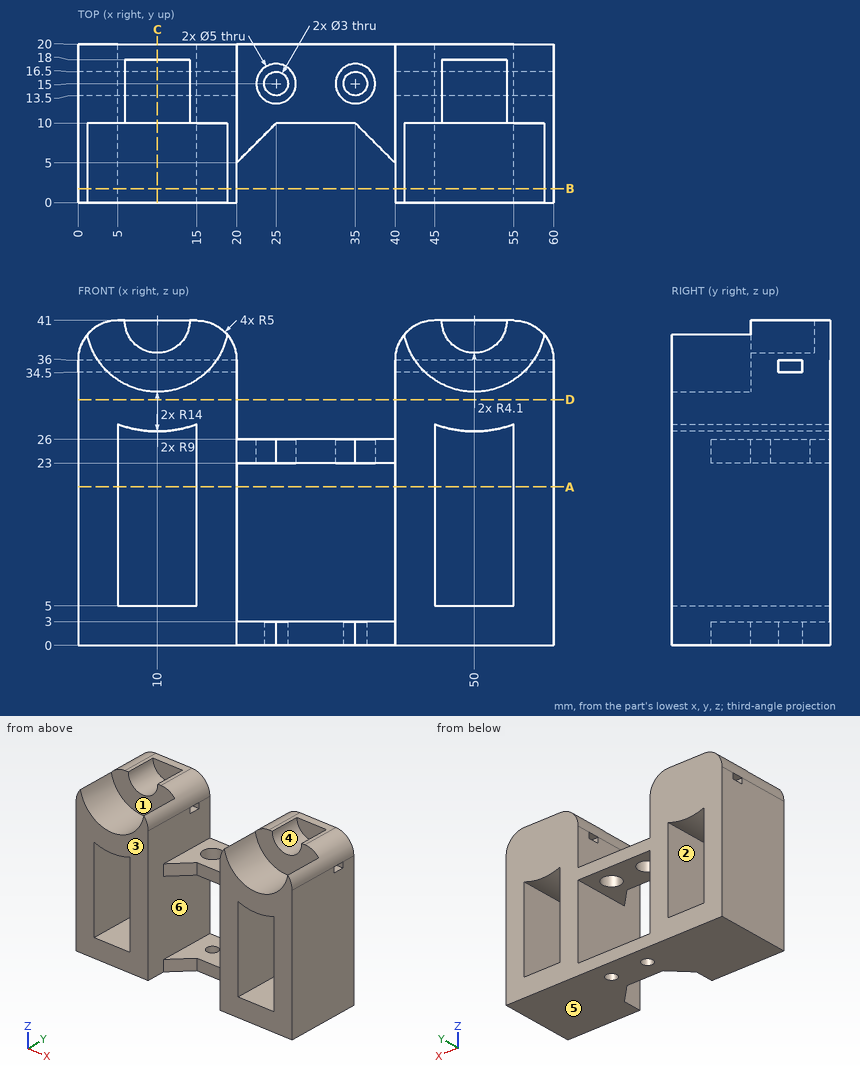
Check sheet for the drawn part. Datum: minimum x, y, z corner. Units: mm. A direction names the side the tool comes from. Round coordinates to 2 decimals unless told otherwise and drop trailing zeros. Loops run counter-clockwise (first coordinate to the right, second up) from the corner with the lowest first, then second, coordinate; pieces in that order, holes last. Notation, with made-up numbers: (71, 24.25) -> (80, 24.25) arc R23 ccw to (80, 57.25) -> close; hole circle Ø10 at (-35, -40). An arc over 180 degrees is marked (long way). Put each result on its own line as item: value. Start each with the question number.
1. Section check B-B (y = 1.75). Enter the section's corners in (x, z).
2. Section check D-D (z = 31). Enter the section's corners in (x, y).
3. Section check C-C (x = 10). Enter the section's corners in (y, z).
4. Gauge pin test, flat ends, axial feed: pin 1 (6 mm diameter, centred on x = 12, z = 28, fed in from -Y); pin 2 (3.5 mm diameter, centred on x = 32, z = 25, fed in from -Y); pin 3 (6.5 mm diameter, centred on x = 35, y = 15, fed in from +Z); pin 4 (1.2 mm diameter, centred on x = 10, z = 40, fed in from -Y). Record the tip position at first contact, or that the pin passes through.
5. Scan lines: probe 1 along X at (y, z) = (6.25, 15); probe 2 along Z at (x, y) = (39.5, 15.5); probe 3 along X at (y, z) = (8.25, 29). Record each from-to range of solid material in increasing order.
6. Section check A-A (z = 20). Enter the section's corners in (x, y), plus the area to 3 significant figures.
7. Access from +Z, -Z, +X, -X, +Y, -Y to the whole of each face (thin tool, end or side, straight path). Record for the marked faces 1, 2 and 3.
8. Draft check along Z on the marked faces 4, 5 and 6. Enter one of: +Z half, -Z half, draft (parallel to the pull), parting line (faces both ways), or undercut.
Findings:
1. outline: (0, 0) -> (20, 0) -> (20, 36) arc R5 ccw to (18.82, 39.22) arc R9 cw to (1.18, 39.22) arc R5 ccw to (0, 36) -> close; (40, 0) -> (60, 0) -> (60, 36) arc R5 ccw to (58.82, 39.22) arc R9 cw to (41.18, 39.22) arc R5 ccw to (40, 36) -> close; hole (5, 5) -> (15, 5) -> (15, 27.92) arc R14 cw to (5, 27.92) -> close; hole (45, 5) -> (55, 5) -> (55, 27.92) arc R14 cw to (45, 27.92) -> close
2. outline: (0, 0) -> (20, 0) -> (20, 20) -> (0, 20) -> close; (40, 0) -> (60, 0) -> (60, 20) -> (40, 20) -> close
3. outline: (0, 0) -> (20, 0) -> (20, 5) -> (0, 5) -> close; (0, 27) -> (20, 27) -> (20, 41) -> (18, 41) -> (18, 36.9) -> (10, 36.9) -> (10, 32) -> (0, 32) -> close; hole (13.5, 34.5) -> (16.5, 34.5) -> (16.5, 36) -> (13.5, 36) -> close
4. pin 1: stops at y = 0
4. pin 2: stops at y = 10
4. pin 3: stops at z = 26
4. pin 4: stops at y = 18
5. probe 1: x = 0 to 5, 15 to 20, 40 to 45, 55 to 60
5. probe 2: z = 0 to 3, 23 to 26
5. probe 3: x = 0 to 20, 40 to 60
6. outline: (0, 0) -> (5, 0) -> (5, 20) -> (0, 20) -> close; (15, 0) -> (20, 0) -> (20, 20) -> (15, 20) -> close; (40, 0) -> (45, 0) -> (45, 20) -> (40, 20) -> close; (55, 0) -> (60, 0) -> (60, 20) -> (55, 20) -> close
6. area: 400 mm^2
7. face 1: +Z, -Y
7. face 2: +Y, -Y
7. face 3: +Z, -Z, +X, -X, -Y
8. face 4: +Z half
8. face 5: -Z half
8. face 6: undercut
